For this review, take the finished solid that the model builds, in its own axes (mm). Give positions to 0.01 mm unless a question says otherwise; leave off trailing zeros. One line per question, with ' | ' between items. Start each with the question number.
(1) Insertion check: P1, Ø3, axis at x = 92.075, y = -19.304, coming from the +Z side; P2, Ø3.5, axis at x = -114.3, z = 4.8, coming from the +Y side. Each pin has a flat end and moves straight along its axis. Give the tip position at first contact, or say it passes through.
(2) Wall thickness on probe 1 along X at (y, z) = (-3, 5.25); probe 2 along Z at (x, y) = (-114.3, -6.75); probe 3 along X at (y, z) = (-20, 6): over which ranges is each line inside the solid? List them lowest first.
(3) Draft analysis for pull direction Y (two halves, no side actions). For faces 1 (the flat face through (-2, -31, 0)), 2 (the cylindrical face through (-119.673, -46.821, 4.733)), 3 (the flat face through (-2, -62.992, 5)), 4 (the flat face through (-2, 0, 5)), state which applies: +Y half, -Y half, draft (parallel to the pull), parting line (faces both ways), or undercut.
from build123d import *

# Parameters (mm, degrees)
SKETCH1_W                        = 266.7
SKETCH1_H                        = 62.992
BOSS_EXTRUDE1_DEPTH              = 9.6012
F_10_32_TAPPED_HOLE1_AT_2_COUNT  = 2
F_10_32_TAPPED_HOLE1_AT_2_PITCH  = 92.075
F_10_32_TAPPED_HOLE1_AT_3_COUNT  = 2
F_10_32_TAPPED_HOLE1_AT_3_PITCH  = 184.15
F_3_8_0_3750_DOWEL_HOLE1_D       = 9.525
F_10_32_TAPPED_HOLE2_D           = 4.0386
F_10_32_TAPPED_HOLE2_DEPTH       = 19.05
F_10_32_TAPPED_HOLE2_CSINK_D     = 5.334
F_10_32_TAPPED_HOLE2_CSINK_ANGLE = 90
F_10_32_TAPPED_HOLE2_TIP         = 1.213317848


with BuildPart() as part:
    # Sketch1 → Boss-Extrude1 (new body)
    with BuildSketch(Plane.XY):
        with Locations((0, -31.496)):
            Rectangle(SKETCH1_W, SKETCH1_H)
    extrude(amount=BOSS_EXTRUDE1_DEPTH)

    # Sketch2 → #10-32 Tapped Hole1 (revolve, cut)
    with BuildSketch(Plane(origin=(92.075, -19.304, 9.6012), x_dir=(0, -1, 0), z_dir=(1, 0, 0))):
        Polygon((0, 0), (0, 9.6012), (2.667, 9.6012), (2.0193, 8.9535), (2.0193, 0.6477), (2.667, 0), align=None)
    f_10_32_tapped_hole1 = revolve(axis=Axis((92.075, -19.304, 15.9512), (0, 0, -1)), mode=Mode.SUBTRACT)

    # #10-32 Tapped Hole1 at 2: #10-32 Tapped Hole1 ×2
    with Locations(*[(-i * F_10_32_TAPPED_HOLE1_AT_2_PITCH, 0, 0) for i in range(1, F_10_32_TAPPED_HOLE1_AT_2_COUNT)]):
        add(f_10_32_tapped_hole1, mode=Mode.SUBTRACT)

    # #10-32 Tapped Hole1 at 3: #10-32 Tapped Hole1 ×2
    with Locations(*[(-i * F_10_32_TAPPED_HOLE1_AT_3_PITCH, 0, 0) for i in range(1, F_10_32_TAPPED_HOLE1_AT_3_COUNT)]):
        add(f_10_32_tapped_hole1, mode=Mode.SUBTRACT)

    # 3/8 (0.3750) Dowel Hole1 (through all)
    with Locations(Plane.XY.offset(9.6012)):
        with Locations((-117.475, -42.5958)):
            Hole(F_3_8_0_3750_DOWEL_HOLE1_D / 2)

    # #10-32 Tapped Hole2
    with Locations(Plane(origin=(0, 0, 0), x_dir=(1, 0, 0), z_dir=(0, 1, 0))):
        with Locations((114.3, -4.8006), (57.15, -4.8006), (-57.15, -4.8006), (-114.3, -4.8006)):
            CounterSinkHole(F_10_32_TAPPED_HOLE2_D / 2, F_10_32_TAPPED_HOLE2_CSINK_D / 2, depth=F_10_32_TAPPED_HOLE2_DEPTH, counter_sink_angle=F_10_32_TAPPED_HOLE2_CSINK_ANGLE)
            with Locations((0, 0, -(F_10_32_TAPPED_HOLE2_DEPTH + F_10_32_TAPPED_HOLE2_TIP / 2))):  # 118° drill point
                Cone(0, F_10_32_TAPPED_HOLE2_D / 2, F_10_32_TAPPED_HOLE2_TIP, mode=Mode.SUBTRACT)


solid = part.part
A:
1) P1: passes through | P2: stops at y = -19.21
2) probe 1: x = -133.35 to -116.27, -112.33 to -59.12, -55.18 to 55.18, 59.12 to 112.33, 116.27 to 133.35 | probe 2: z = 0 to 2.78, 6.82 to 9.6 | probe 3: x = -133.35 to -93.97, -90.18 to -1.9, 1.9 to 90.18, 93.97 to 133.35
3) face 1: draft | face 2: undercut | face 3: -Y half | face 4: +Y half
